Autodesk Inventor part; units mm, degrees
ref_plane "Work Plane1" through (0, 8, 0) normal (0, 1, 0) x (1, 0, 0)
ref_plane "YZ Plane" through (0, 0, 0) normal (1, 0, 0) x (0, 1, 0)
ref_plane "XZ Plane" through (0, 0, 0) normal (0, 1, 0) x (-1, 0, 0)
sketch "Sketch1" plane through (0, 0, 0) normal (0, 1, 0) x (-1, 0, 0)
  arc A0 (31.569, 13.7227) -> (30.069, 12.2227) centre (31.569, 12.2227) ccw
  line L0 (31.569, 13.7227) -> (34.069, 13.7227)
  line L1 (34.069, 13.7227) -> (34.069, 18.9227)
  line L2 (32.069, 20.9227) -> (2.569, 20.9227)
  line L3 (34.069, -13.2773) -> (31.569, -13.2773)
  arc A1 (30.069, -11.7773) -> (31.569, -13.2773) centre (31.569, -11.7773) ccw
  arc A2 (34.069, 18.9227) -> (32.069, 20.9227) centre (32.069, 18.9227) ccw
  arc A3 (34.0195, 22.4149) -> (32.069, 23.9727) centre (32.069, 21.9727) ccw
  line L4 (32.069, 23.9727) -> (-23.931, 23.9727)
  arc A4 (-23.931, 23.9727) -> (-25.931, 21.9727) centre (-23.931, 21.9727) ccw
  line L5 (-25.931, 21.9727) -> (-25.931, -21.0273)
  arc A5 (-25.931, -21.0273) -> (-23.931, -23.0273) centre (-23.931, -21.0273) ccw
  line L6 (-23.931, -23.0273) -> (32.069, -23.0273)
  arc A6 (32.069, -23.0273) -> (33.899, -21.8341) centre (32.069, -21.0273) ccw
  arc A7 (32.069, -20.2773) -> (34.069, -18.2773) centre (32.069, -18.2773) ccw
  line L7 (32.069, -20.2773) -> (0.569, -20.2773)
  line L8 (34.069, -13.2773) -> (34.069, 13.7227)
  line L9 (0.569, -22.2773) -> (0.569, 18.9227)
  line L10 (30.069, -11.7773) -> (30.069, 12.2227)
  line L11 (34.069, -18.2773) -> (34.069, -13.2773)
  line L12 (2.569, 22.9227) -> (32.069, 22.9227)
  line L13 (0.569, -22.2773) -> (32.069, -22.2773)
  arc A8 (32.069, -22.2773) -> (36.069, -18.2773) centre (32.069, -18.2773) ccw
  line L14 (36.069, -18.2773) -> (36.069, 18.9227)
  arc A9 (2.569, 20.9227) -> (0.569, 18.9227) centre (2.569, 18.9227) ccw
  line L15 (-1.431, 14.4227) -> (-1.431, 18.9227)
  arc A10 (2.569, 22.9227) -> (-1.431, 18.9227) centre (2.569, 18.9227) ccw
  arc A11 (36.069, 18.9227) -> (32.069, 22.9227) centre (32.069, 18.9227) ccw
  line L16 (-1.431, 14.4227) -> (0.569, 14.4227)
  point P0 (0.569, 20.9227)
  dimension "d8" = 2
  dimension "d9" = 2
  dimension "d66" = 2
  dimension "d67" = 2
  dimension "d68" = 4.5
  dimension "d69" = 4
extrude "Extrusion3" add sketch "Sketch1" against normal blind 2 contours L0 L8 L3 A1 L10 A0 | A0 L10 A1 L3 L11 A7 L7 L9 A9 L2 A2 L1 L0 | L1 A2 L2 A9 L9 L16 L15 A10 L12 A11 L14 A8 L13 L7 A7 L11 L8
ref_plane "Work Plane1" through (0, 8, 0) normal (0, 1, 0) x (1, 0, 0)
extrude "Extrusion4" add sketch "Sketch1" along normal blind 8 contours L1 A2 L2 A9 L9 L16 L15 A10 L12 A11 L14 A8 L13 L7 A7 L11 L8
sketch "Sketch2" plane through (0, 8, 0) normal (0, 1, 0) x (1, 0, 0)
  line L0 (23.931, 23.0273) -> (-32.069, 23.0273)
  arc A0 (-32.069, 23.0273) -> (-33.899, 21.8341) centre (-32.069, 21.0273) ccw
  line L1 (-32.069, -23.9727) -> (23.931, -23.9727)
  arc A1 (-34.0195, -22.4149) -> (-32.069, -23.9727) centre (-32.069, -21.9727) ccw
  arc A2 (-32.069, 23.0273) -> (-34.069, 21.0273) centre (-32.069, 21.0273) ccw
  arc A3 (-34.069, -21.9727) -> (-32.069, -23.9727) centre (-32.069, -21.9727) ccw
  line L2 (-34.069, 18.2773) -> (-34.069, 13.2773)
  line L3 (-34.069, 13.2773) -> (-34.069, -13.7227)
  line L4 (-34.069, -13.7227) -> (-34.069, -18.9227)
  line L5 (-34.069, -21.9727) -> (-34.069, 21.0273)
  arc A4 (-32.069, 25.0273) -> (-36.069, 21.0273) centre (-32.069, 21.0273) ccw
  line L6 (-0.569, 25.0273) -> (-32.069, 25.0273)
  line L7 (-0.569, -25.9727) -> (-32.069, -25.9727)
  line L8 (-0.569, -23.9727) -> (-0.569, -25.9727)
  line L9 (-0.569, 20.2773) -> (-0.569, 25.0273)
  line L10 (-0.569, 22.2773) -> (-0.569, 22.2773)
  line L11 (-32.069, 23.0273) -> (-0.569, 23.0273)
  line L12 (-32.069, -23.9727) -> (-0.569, -23.9727)
  line L13 (-32.069, -20.9227) -> (-2.569, -20.9227)
  line L14 (-0.569, -14.4227) -> (-0.569, 20.2773)
  line L15 (-0.569, 20.2773) -> (-32.069, 20.2773)
  arc A5 (-32.069, 20.2773) -> (-34.069, 18.2773) centre (-32.069, 18.2773) ccw
  line L16 (-34.069, 18.2773) -> (-34.069, -18.9227)
  arc A6 (-34.069, -18.9227) -> (-32.069, -20.9227) centre (-32.069, -18.9227) ccw
  line L17 (-32.069, 22.2773) -> (-0.569, 22.2773)
  line L18 (-0.569, 22.2773) -> (-0.569, 22.2773)
  arc A7 (-2.569, -20.9227) -> (-0.569, -18.9227) centre (-2.569, -18.9227) ccw
  line L19 (-0.569, -18.9227) -> (-0.569, -14.4227)
  line L20 (-0.569, -23.9727) -> (-0.569, -18.9227)
  line L21 (-36.069, 21.0273) -> (-36.069, -21.9727)
  arc A8 (-36.069, -21.9727) -> (-32.069, -25.9727) centre (-32.069, -21.9727) ccw
  point P0 (0, 0)
  point P1 (-32.069, 25.0273)
  dimension "d19" = 2
  dimension "d20" = 2
  dimension "d21" = 31.5
  dimension "d22" = 31.5
  dimension "d23" = 31.5
extrude "Extrusion7" add sketch "Sketch2" against normal blind 2 contours L9 L15 A5 L5 A2 A0 L0 | L0 A0 A2 L5 L2 L3 L4 A3 A1 L1 L8 L7 A8 L21 A4 L6 L9 | L20 L1 A1 A3 L5 A6 L13 A7
extrude "Extrusion8" add sketch "Sketch2" along normal blind 15 contours L0 A0 A2 L5 L2 L3 L4 A3 A1 L1 L8 L7 A8 L21 A4 L6 L9
sketch "Sketch5" plane through (0, 23, 0) normal (0, 1, 0) x (1, 0, 0)
  circle A0 centre (-17.319, 30.0273) radius 5
  circle A1 centre (-17.319, 30.0273) radius 3
  arc A2 (-12.4777, 28.7773) -> (-9.573, 25.0273) centre (-9.573, 28.0273) ccw
  arc A3 (-25.0649, 25.0273) -> (-22.1602, 28.7773) centre (-25.0649, 28.0273) ccw
  line L0 (-0.569, 23.0273) -> (-0.569, 25.0273)
  circle A4 centre (-6.0917, -30.9727) radius 5
  circle A5 centre (-6.0917, -30.9727) radius 2.5
  arc A6 (-10.305, -28.2804) -> (-11.569, -25.9727) centre (-11.569, -27.4727) ccw
  arc A7 (-0.6145, -25.9727) -> (-1.8785, -28.2804) centre (-0.6145, -27.4727) ccw
  circle A8 centre (-26.5917, -30.9727) radius 5
  circle A9 centre (-26.5917, -30.9727) radius 2.5
  arc A10 (-30.805, -28.2804) -> (-32.069, -25.9727) centre (-32.069, -27.4727) ccw
  arc A11 (-21.1145, -25.9727) -> (-22.3785, -28.2804) centre (-21.1145, -27.4727) ccw
  line L1 (-0.569, -25.9727) -> (-0.569, -23.9727)
  line L2 (-0.569, 25.0273) -> (-32.069, 25.0273)
  line L3 (-32.069, -25.9727) -> (-0.569, -25.9727)
  point P0 (0, 0)
  point P1 (1.0185, -24.3852)
  point P2 (-26.5917, -25.9727)
  point P3 (-6.0917, -25.9727)
  point P4 (-17.319, 25.0273)
  dimension "d34" = 10
  dimension "d35" = 6
  dimension "d38" = 3
  dimension "d39" = 3
  dimension "d40" = 10
  dimension "d41" = 5
  dimension "d42" = 3
  dimension "d43" = 3
  dimension "d44" = 10
  dimension "d45" = 5
  dimension "d46" = 3
  dimension "d47" = 3
  dimension "d49" = 20.5
extrude "Extrusion10" add sketch "Sketch5" against normal blind 2
sketch "Sketch6" plane through (0, -2, 0) normal (0, -1, 0) x (1, 0, 0)
  line L0 (-0.569, -22.2773) -> (-0.569, 14.4227)
  line L1 (-2.569, 22.9227) -> (-32.069, 22.9227)
  arc A0 (-32.069, 22.9227) -> (-36.069, 18.9227) centre (-32.069, 18.9227) ccw
  line L2 (-36.069, 18.9227) -> (-36.069, -18.2773)
  arc A1 (-36.069, -18.2773) -> (-32.069, -22.2773) centre (-32.069, -18.2773) ccw
  line L3 (-32.069, -22.2773) -> (-0.569, -22.2773)
  line L4 (-30.069, 18.9227) -> (-6.569, 18.9227)
  line L5 (-4.569, 16.9227) -> (-4.569, -16.2773)
  line L6 (-6.569, -18.2773) -> (-30.069, -18.2773)
  line L7 (-32.069, -16.2773) -> (-32.069, 16.9227)
  arc A2 (-6.569, -18.2773) -> (-4.569, -16.2773) centre (-6.569, -16.2773) ccw
  arc A3 (-32.069, -16.2773) -> (-30.069, -18.2773) centre (-30.069, -16.2773) ccw
  arc A4 (-30.069, 18.9227) -> (-32.069, 16.9227) centre (-30.069, 16.9227) ccw
  arc A5 (-4.569, 16.9227) -> (-6.569, 18.9227) centre (-6.569, 16.9227) ccw
  line L8 (-0.569, 14.4227) -> (1.431, 14.4227)
  line L9 (1.431, 14.4227) -> (1.431, 18.9227)
  arc A6 (1.431, 18.9227) -> (-2.569, 22.9227) centre (-2.569, 18.9227) ccw
  point P0 (0, 0)
  point P1 (-4.569, 18.9227)
  point P2 (-4.569, -18.2773)
  dimension "d52" = 4
  dimension "d53" = 37.2
  dimension "d54" = 27.5
  dimension "d55" = 4
  dimension "d56" = 2
extrude "Extrusion11" cut sketch "Sketch6" against normal blind 2 contours L4 A5 L5 A2 L6 A3 L7 A4
sketch "Sketch7" plane through (-36.069, -2, -18.2773) normal (-1, 0, 0) x (0, 0, 1)
  line L0 (2.75, 25) -> (34.75, 25)
  line L1 (34.75, 25) -> (34.75, 17)
  line L2 (32.75, 15) -> (4.75, 15)
  line L3 (2.75, 17) -> (2.75, 25)
  arc A0 (2.75, 17) -> (4.75, 15) centre (4.75, 17) ccw
  arc A1 (32.75, 15) -> (34.75, 17) centre (32.75, 17) ccw
  point P0 (18.2773, 2)
  point P1 (40.25, 25)
  point P2 (-2.75, 25)
  point P3 (34.75, 21)
  point P4 (40.25, 8)
  dimension "d59" = 2
  dimension "d61" = 32
  dimension "d62" = 43
extrude "Extrusion12" cut sketch "Sketch7" against normal blind 6
sketch "Sketch8" plane through (0, 8, 0) normal (0, 1, 0) x (1, 0, 0)
  line L0 (-0.569, -14.4227) -> (-0.569, -18.9227)
  line L1 (1.431, -14.4227) -> (-0.569, -14.4227)
  line L2 (1.431, -18.9227) -> (1.431, -14.4227)
  arc A0 (-0.569, -22.3868) -> (1.431, -18.9227) centre (-2.569, -18.9227) ccw
  line L3 (-0.569, -23.9727) -> (-0.569, -18.9227)
  point P0 (0, 0)
extrude "Extrusion13" cut sketch "Sketch8" against normal blind 6
properties part number "CO-1-01-motorControllersMount"
Part model, mm, in its own coordinate system. A direction names the side the tool comes from. Coordinates: 2 decimals unless noted, no trailing zeros. Write each loop counter-clockwise with the first axis right and the second up, starting at its lowest first coordinate (ties: lowest second). Pieces come first, ordered by that corner, then holes. Notation, with made-up numbers: (89.5, 83) - (120.5, 83) arc R20 cw to (120.5, 100) - close; hole circle Ø5 at (3, 24.5). An arc over 180 degrees is marked (long way). Put each result on its own line as item: value.
1. 3-axis set-ups, long thin cutter, end or side, ignore diameter. For faces 1 (the flat face through (-24, 21, 30)), 2 (the cylindrical face through (-33.175, 15.395, -22.694)), 3 (the flat face through (-35, 19, -15.527)): which of +Z, -Z, +X, -X, +Y, -Y reach the whole face in a straight line?
Final values:
face 1: +Z, +X, -X, -Y
face 2: +X, +Y
face 3: +X, -X, +Y
2. Band-saw the part on C-C (x = -5.5). Write the cut outline in (y, z), then the cut area to 3 significant figures.
Final values:
outline: (-2, -22.28) - (6, -22.28) - (6, -25.03) - (23, -25.03) - (23, -23.03) - (8, -23.03) - (8, -20.28) - (0, -20.28) - (0, -17.97) - (-2, -17.97) - close; (-2, 18.61) - (0, 18.61) - (0, 20.92) - (8, 20.92) - (8, 23.97) - (23, 23.97) - (23, 28.54) - (21, 28.54) - (21, 25.97) - (6, 25.97) - (6, 22.92) - (-2, 22.92) - close; (21, 33.4) - (23, 33.4) - (23, 35.94) - (21, 35.94) - close
area: 131 mm²
3. Two-plate mould, pull along Z, no slides. Class faces 4 (the flat face through (-17, 15, 23.973)), 5 (the flat face through (-35, 19, 16.473)), 6 (the flat face through (-0.569, 10, 25)), 7 (the flat face through (0, 0, 14.423)): +Z half, -Z half, draft (parallel to the pull), parting line (faces both ways), or undercut.
Final values:
face 4: undercut
face 5: undercut
face 6: draft
face 7: -Z half
4. Band-saw the part on D-D (x = -13.5). Write the cut outline in (y, z), then the cut area to 3 significant figures.
Final values:
outline: (-2, -22.28) - (6, -22.28) - (6, -25.03) - (21, -25.03) - (21, -33.25) - (23, -33.25) - (23, -23.03) - (8, -23.03) - (8, -20.28) - (0, -20.28) - (0, -18.28) - (-2, -18.28) - close; (-2, 18.92) - (0, 18.92) - (0, 20.92) - (8, 20.92) - (8, 23.97) - (23, 23.97) - (23, 25.97) - (6, 25.97) - (6, 22.92) - (-2, 22.92) - close
area: 136 mm²
5. Probe line 1 along Z through (x, y) = (-14, 13); line 2 along Z through (x, y) = (-10.5, 5); line 3 along X through (y, z) = (4.5, -4.5). List the from-to ranges inside material, lowest first. Write a range as [from, to].
Final values:
line 1: z = [-25.03, -23.03], [23.97, 25.97]
line 2: z = [-22.28, -20.28], [20.92, 22.92]
line 3: x = [-36.07, -34.07]
6. Flat gauge pins, fed straight in: pin 1 Ø1.6 at (x, z) = (-35, 0.5) entering from +Y; pin 2 Ø4 at (x, z) = (-15, -20.5) entering from +Y; pin 3 Ø12.5 at (y, z) = (8, -0.5) entering from +X; pin 4 Ø3 at (x, z) = (-18.5, -30.5) entering from -Y. Where does each tip first touch, or does it go through?
Final values:
pin 1: stops at y = 13
pin 2: stops at y = 8
pin 3: stops at x = -34.07
pin 4: passes through
7. Band-saw the part on B-B (y = 11.25). Write the cut outline in (x, z), then the cut area to 3 significant figures.
Final values:
outline: (-36.07, -21.03) arc R4 ccw to (-32.07, -25.03) - (-0.57, -25.03) - (-0.57, -23.03) - (-32.07, -23.03) arc R2 cw to (-33.9, -21.83) arc R2 cw to (-34.07, -21.03) - (-34.07, 21.97) arc R2 cw to (-34.02, 22.41) arc R2 cw to (-32.07, 23.97) - (-0.57, 23.97) - (-0.57, 25.97) - (-32.07, 25.97) arc R4 ccw to (-36.07, 21.97) - close
area: 231 mm²
8. Band-saw the part on A-A (z = -11). Write the cut outline in (x, y), then the cut area to 3 significant figures.
Final values:
outline: (-36.07, -2) - (-32.07, -2) - (-32.07, 0) - (-34.07, 0) - (-34.07, 13) - (-36.07, 13) - close; (-4.57, -2) - (-0.57, -2) - (-0.57, 0) - (-4.57, 0) - close
area: 42.0 mm²
